from build123d import *

# Parameters (mm, degrees)
SKETCH1_R           = 1.5
BOSS_EXTRUDE1_DEPTH = 3


with BuildPart() as part:
    # Sketch1 → Boss-Extrude1 (new body)
    with BuildSketch(Plane.XY):
        with BuildLine():
            ThreePointArc((-105.112423116, -13.831138676), (-96.691314892, 2.069847591), (-79.69956033, 7.989028691))
            Line((-79.69956033, 7.989028691), (-68.289776062, 7.543112506))
            ThreePointArc((-68.289776062, 7.543112506), (-56.37401605, 8.503345495), (-45.024076574, 12.256511885))
            ThreePointArc((-45.024076574, 12.256511885), (-32.132147942, 14.423979547), (-19.981968964, 9.599781095))
            ThreePointArc((-19.981968964, 9.599781095), (-14.269337445, 8.685833715), (-18.71157232, 12.392045797))
            ThreePointArc((-18.71157232, 12.392045797), (-32.153587478, 17.440965919), (-46.2987226, 14.9722581))
            ThreePointArc((-46.2987226, 14.9722581), (-56.969685192, 11.443613896), (-68.172619764, 10.540824034))
            Line((-68.172619764, 10.540824034), (-79.582404032, 10.986740218))
            ThreePointArc((-79.582404032, 10.986740218), (-98.709612397, 4.290845071), (-108.111857285, -13.661394421))
            ThreePointArc((-108.111857285, -13.661394421), (-106.928371833, -19.334178574), (-105.112423116, -13.831138676))
        make_face()
        with Locations((-106.758866773, -16.338971063)):
            Circle(SKETCH1_R, mode=Mode.SUBTRACT)
        with Locations((-17, 9.92820323)):
            Circle(SKETCH1_R, mode=Mode.SUBTRACT)
    extrude(amount=BOSS_EXTRUDE1_DEPTH)


solid = part.part
Verification items for the finished model (mm, model axes). A direction names the side the tool comes from. Round coordinates to 2 decimals unless told otherwise and drop trailing zeros. Order: outer loops, then holes, each group sorted by start corner. A loop starts at its lowest first (then second) coordinate and runs counter-clockwise, first axis right, second up. Notation, with made-up numbers: (87, 78.25) -> (127, 78.25) arc R29 cw to (127, 101.25) -> close; hole circle Ø11 at (89, -32.75). An arc over 180 degrees is marked (long way). Put each result on its own line as item: value.
1) Section check C-C (y = -10). Record the cut outline in (x, z), then the cut area to 3 significant figures.
Final values:
outline: (-107.47, 0) -> (-104.37, 0) -> (-104.37, 3) -> (-107.47, 3) -> close
area: 9.30 mm^2
2) Section check D-D (x = -89.5). Record the cut outline in (y, z).
Final values:
outline: (6.37, 0) -> (9.55, 0) -> (9.55, 3) -> (6.37, 3) -> close
3) Mould release check, pull along X, two halves, no side actions. Record for faces 1 (the cylindrical face through (-107.038, -19.326, 1.479)), 2 (the flat face through (-66, 9, 0)), 3 (the cylindrical face through (-96.89, 1.9, 1.48)): +X half, -X half, draft (parallel to the pull), parting line (faces both ways), or undercut.
Final values:
face 1: parting line
face 2: draft
face 3: undercut
4) Section check B-B (z = 0.7). Record the cut outline in (x, y).
Final values:
outline: (-108.11, -13.66) arc R3 ccw (long way) to (-105.11, -13.83) arc R24.61 cw to (-79.7, 7.99) -> (-68.29, 7.54) arc R50.15 ccw to (-45.02, 12.26) arc R24.31 cw to (-19.98, 9.6) arc R3 ccw (long way) to (-18.71, 12.39) arc R27.31 ccw to (-46.3, 14.97) arc R47.15 cw to (-68.17, 10.54) -> (-79.58, 10.99) arc R27.61 ccw to start; hole circle Ø3 at (-106.76, -16.34); hole circle Ø3 at (-17, 9.93)
5) Set-up check for faces 4 (the cylindrical face through (-18.5, 10, 1.5)), 5 (the flat face through (-73.8, 10.76, 1.48)), 6 (the cylindrical face through (-56.54, 8.47, 1.48)): record each of +Z, -Z, +X, -X, +Y, -Y from which the full face is reachable in a straight line by a thin tool's end or side.
Final values:
face 4: +Z, -Z
face 5: +Z, -Z, +Y
face 6: +Z, -Z, -Y
6) Material ranges on line 1 (Y direction, x = -17, z = 1.65); line 2 (Y direction, x = -67, z = 1.05); line 3 (X direction, y = -0.5, z = 0.65), recorded low to high.
Final values:
line 1: y = 6.93 to 8.43, 11.43 to 12.93
line 2: y = 7.51 to 10.51
line 3: x = -103.09 to -99.27
7) Section check A-A (x = -17). Record the cut outline in (y, z), then the cut area to 3 significant figures.
Final values:
outline: (6.93, 0) -> (8.43, 0) -> (8.43, 3) -> (6.93, 3) -> close; (11.43, 0) -> (12.93, 0) -> (12.93, 3) -> (11.43, 3) -> close
area: 9.00 mm^2
